```python
from build123d import *

# Parameters (mm, degrees)
SKETCH1_R           = 2.0828
EXTRUDE1_DEPTH      = 19.05
CHAMFER2_SIZE       = 0.5953125
SKETCH27_R          = 4.7625
BOSS_EXTRUDE4_DEPTH = 4.7625
SKETCH21_R          = 5.3578125
BOSS_EXTRUDE1_DEPTH = 3.96875
CHAMFER3_SIZE       = 0.396875


with BuildPart() as part:
    # Sketch1 → Extrude1 (new body)
    with BuildSketch(Plane.XY):
        Circle(SKETCH1_R)
    extrude(amount=-EXTRUDE1_DEPTH)

    # Chamfer2
    chamfer2_edges = [part.edges().sort_by_distance(p)[0] for p in [
        (-2.0828, 0, -19.05),
    ]]
    chamfer(chamfer2_edges, length=CHAMFER2_SIZE)

    # Sketch27 → Boss-Extrude4 (add)
    with BuildSketch(Plane.XY):
        Circle(SKETCH27_R)
    extrude(amount=BOSS_EXTRUDE4_DEPTH)

    # Sketch21 → Boss-Extrude1 (add)
    with BuildSketch(Plane.XY.offset(4.7625)):
        Circle(SKETCH21_R)
    extrude(amount=BOSS_EXTRUDE1_DEPTH)

    # Sketch28 → Cut-Revolve1 (revolve, cut)
    with BuildSketch(Plane(origin=(0, 0, 0), x_dir=(0, 0, -1), z_dir=(1, 0, 0))):
        with BuildLine():
            Line((-4.7625, 4.7625), (-0.9525, 4.7625))
            ThreePointArc((-0.9525, 4.7625), (-2.8575, 3.442334108), (-4.7625, 4.7625))
        make_face()
    revolve(axis=Axis((0, 0, 0), (0, 0, -1)), mode=Mode.SUBTRACT)

    # Chamfer3
    chamfer3_edges = [part.edges().sort_by_distance(p)[0] for p in [
        (-5.3578125, 0, 4.7625),
        (-5.3578125, 0, 8.73125),
    ]]
    chamfer(chamfer3_edges, length=CHAMFER3_SIZE)


solid = part.part
```
For this review, take the finished solid that the model builds, in its own axes (mm). A direction names the side the tool comes from. Coordinates: 2 decimals unless noted, no trailing zeros. Order: outer loops, then holes, each group sorted by start corner. A loop starts at its lowest first (then second) coordinate and runs counter-clockwise, first axis right, second up. Notation, with made-up numbers: (10, 65.5) - (42, 65.5) arc R22 cw to (42, 88.5) - close; hole circle Ø4 at (70.25, -17). An arc over 180 degrees is marked (long way). Answer as a JSON object with one key per item and string values. Group by question number.
1. We need section D-D on z = -7.5. State the section outline as (x, y) points, then the cut area to 3 significant figures.
2. For faces 1 (the flat face through (2, -1, 0)), 2 (the flat face through (0, 0, 8.731)), list the 3-axis set-ups (+Z, -Z, +X, -X, +Y, -Y) from which the entire face can be reached by the end or side of a thin tool; tool diameter is ignored.
3. We need section C-C on z = 1.5. State the section outline as (x, y) points, then the cut area to 3 significant figures.
4. Clearance check with flat-ended pins moving along their axes: P1, Ø5, axis at x = -0.5, z = 2, coming from the -Y side; P2, Ø6, axis at x = -4, y = 1.5, coming from the -Z side; P3, Ø5, axis at x = -4, y = 3.5, coming from the -Z side; P4, Ø4, axis at x = 3, z = -9, coming from the +Y side. State where each tip first meets the part, or that it passes through.
5. We need section A-A on y = 0. State the section outline as (x, z) points.
6. For probe 1 along Z at (x, y) = (2.5, -1); probe 2 along Z at (x, y) = (3.25, 2.25); probe 3 along Z at (x, y) = (4.75, 0.75), list the stretches that pass through material, from the lowest coordinate up.
Final values:
{
 "1": {"outline": "circle Ø4.17 at (0, 0)", "area": "13.6 mm²"},
 "2": {"face 1": "-Z", "face 2": "+Z, +X, -X, +Y, -Y"},
 "3": {"outline": "circle Ø7.92 at (0, 0)", "area": "49.3 mm²"},
 "4": {"P1": "y = -4.76", "P2": "z = -19.05", "P3": "z = 0", "P4": "y = 1.83"},
 "5": {"outline": "(-5.36, 5.16) - (-4.96, 4.76) - (-4.76, 4.76) arc R2.03 cw to (-4.76, 0.95) - (-4.76, 0) - (-2.08, 0) - (-2.08, -18.45) - (-1.49, -19.05) - (1.49, -19.05) - (2.08, -18.45) - (2.08, 0) - (4.76, 0) - (4.76, 0.95) arc R2.03 cw to (4.76, 4.76) - (4.96, 4.76) - (5.36, 5.16) - (5.36, 8.33) - (4.96, 8.73) - (-4.96, 8.73) - (-5.36, 8.33) - close"},
 "6": {"probe 1": "0 to 8.73", "probe 2": "0 to 1.51, 4.21 to 8.73", "probe 3": "4.76 to 8.73"}
}
